Model file for the job. Use its own axes, mm. Round coordinates to 2 decimals unless told otherwise and drop trailing zeros. Write each loop counter-clockwise with the first axis right and the second up, starting at its lowest first coordinate (ties: lowest second). Pieces come first, ordered by that corner, then holes. Notation, with made-up numbers: (-0.5, -26.75) - (50.5, -26.75) arc R19 cw to (50.5, -1.75) - close; hole circle Ø1 at (-23.75, -36.5). An arc over 180 degrees is marked (long way). One line per item, written item: value.
from build123d import *

# Parameters (mm, degrees)
SKETCH_1_R          = 50
EXTRUDE_1_DEPTH     = 4
SKETCH_2_R          = 1.6
SKETCH_2_R_2        = 5.2
CUT_EXTRUDE_1_DEPTH = 4
SKETCH_3_R          = 1.6
CUT_EXTRUDE_2_DEPTH = 10


with BuildPart() as part:
    # 草图1 → 凸台-拉伸1 (new body)
    with BuildSketch(Plane(origin=(0, 0, 0), x_dir=(1, 0, 0), z_dir=(0, 1, 0))):
        with Locations(Location((0, 0, 0), (0, 0, 270))):
            Circle(SKETCH_1_R)
    extrude(amount=EXTRUDE_1_DEPTH)

    # 草图2 → 切除-拉伸1 (cut)
    with BuildSketch(Plane(origin=(0, 4, 0), x_dir=(1, 0, 0), z_dir=(0, 1, 0))):
        with Locations(Location((0, 8, 0), (0, 0, 270))):
            Circle(SKETCH_2_R)
        with Locations(Location((8, 0, 0), (0, 0, 270))):
            Circle(SKETCH_2_R)
        with Locations(Location((0, -8, 0), (0, 0, 270))):
            Circle(SKETCH_2_R)
        with Locations(Location((-8, 0, 0), (0, 0, 270))):
            Circle(SKETCH_2_R)
        with Locations(Location((0, 0, 0), (0, 0, 270))):
            Circle(SKETCH_2_R_2)
    extrude(amount=-CUT_EXTRUDE_1_DEPTH, mode=Mode.SUBTRACT)

    # 草图3 → 切除-拉伸2 (cut)
    with BuildSketch(Plane(origin=(0, 4, 0), x_dir=(1, 0, 0), z_dir=(0, 1, 0))):
        with Locations(Location((0, 40, 0), (0, 0, 270))):
            Circle(SKETCH_3_R)
        with Locations(Location((23.511410092, 32.360679775, 0), (0, 0, 270))):
            Circle(SKETCH_3_R)
        with Locations(Location((38.042260652, 12.360679775, 0), (0, 0, 270))):
            Circle(SKETCH_3_R)
        with Locations(Location((38.042260652, -12.360679775, 0), (0, 0, 270))):
            Circle(SKETCH_3_R)
        with Locations(Location((23.511410092, -32.360679775, 0), (0, 0, 270))):
            Circle(SKETCH_3_R)
        with Locations(Location((0, -40, 0), (0, 0, 270))):
            Circle(SKETCH_3_R)
        with Locations(Location((-23.511410092, -32.360679775, 0), (0, 0, 270))):
            Circle(SKETCH_3_R)
        with Locations(Location((-38.042260652, -12.360679775, 0), (0, 0, 270))):
            Circle(SKETCH_3_R)
        with Locations(Location((-38.042260652, 12.360679775, 0), (0, 0, 270))):
            Circle(SKETCH_3_R)
        with Locations(Location((-23.511410092, 32.360679775, 0), (0, 0, 270))):
            Circle(SKETCH_3_R)
    extrude(amount=-CUT_EXTRUDE_2_DEPTH, mode=Mode.SUBTRACT)


solid = part.part
1. Drop a flat-ended pin along its axis: pin 1 (2 mm diameter, centred on x = -3, y = 1, fed in from +Z). Give the stop position or say it passes through.
Report:
pin 1: z = 49.96
2. Wall check: probe 1 along X at (y, z) = (2.6, 0); probe 2 along Z at (x, y) = (37.5, 1.9); probe 3 along X at (y, z) = (1.2, -0.5). Give the ranges that are in metal, low to high. Write a range as [from, to].
Report:
probe 1: [-50, -9.6], [-6.4, -5.2], [5.2, 6.4], [9.6, 50]
probe 2: [-33.07, -13.87], [-10.86, 10.86], [13.87, 33.07]
probe 3: [-50, -9.52], [-6.48, -5.18], [5.18, 6.48], [9.52, 50]
3. Band-saw the part on B-B on x = 0. Write the cut outline in (y, z), plus the area to 3 significant figures.
Report:
outline: (0, -50) - (4, -50) - (4, -41.6) - (0, -41.6) - close; (0, -38.4) - (4, -38.4) - (4, -9.6) - (0, -9.6) - close; (0, -6.4) - (4, -6.4) - (4, -5.2) - (0, -5.2) - close; (0, 5.2) - (4, 5.2) - (4, 6.4) - (0, 6.4) - close; (0, 9.6) - (4, 9.6) - (4, 38.4) - (0, 38.4) - close; (0, 41.6) - (4, 41.6) - (4, 50) - (0, 50) - close
area: 307 mm²
4. Band-saw the part on A-A on z = 40. Write the cut outline in (x, y).
Report:
outline: (-30, 0) - (-1.6, 0) - (-1.6, 4) - (-30, 4) - close; (1.6, 0) - (30, 0) - (30, 4) - (1.6, 4) - close
5. Band-saw the part on C-C on z = 0. Write the cut outline in (x, y), plus the area to 3 significant figures.
Report:
outline: (-50, 0) - (-9.6, 0) - (-9.6, 4) - (-50, 4) - close; (-6.4, 0) - (-5.2, 0) - (-5.2, 4) - (-6.4, 4) - close; (5.2, 0) - (6.4, 0) - (6.4, 4) - (5.2, 4) - close; (9.6, 0) - (50, 0) - (50, 4) - (9.6, 4) - close
area: 333 mm²
6. Band-saw the part on D-D on y = 0.8. State how many separate pieces and enclosed holes the cut face has, plus the area to 3 significant figures.
Report:
separate pieces: 1
enclosed holes: 15
area: 7,660 mm²
7. Mould opens along X. For faces 1 (the face through (1.56, 2.03, 4.96)), 2 (the face through (15.02, 1.97, 47.69)), 3 (the face through (-10, 0, -1)) say: released by +X, released by -X, zero draft, split by the parting line, or undercut.
Report:
face 1: undercut
face 2: split by the parting line
face 3: zero draft
